The model under review builds one solid part; all positions refer to its coordinate system, in mm. Give positions to 0.01 mm unless a question says otherwise; leave off trailing zeros. Loops run counter-clockwise (first coordinate to the right, second up) from the corner with the lowest first, then second, coordinate; pieces in that order, holes last. Notation, with made-up numbers: M 65.5,37 L 122.5,37 A20 ccw 122.5,62 Z; hole C 81.5,52.5 d6. An arc over 180 degrees is marked long. One line per item, written item: value. Start each with the question number.
Q1. We need section B-B on z = -15377.5. Write out the cut boundary in (x, y).
Q2. To check wall thickness, follow line 1 along Z through (x, y) = (-9686, 2.5); line 2 along Z through (x, y) = (-9702, 3.1); line 3 along X through (y, z) = (2.9, -15375). State the ranges of each line that lie inside material, in increasing order. Write a range as from..to.
Q3. We need section A-A on y = 2.75. Write out the cut boundary in (x, z), plus the area to 3 significant figures.
Q4. We need section C-C on z = -15394. Write out the cut boundary in (x, y).
Q5. For pin 1 (1 mm diameter, centred on y = 2, z = -15392.5, fed in from +X); pin 2 (2 mm diameter, centred on x = -9630, y = 1.5, fed in from +Z), all flat-tipped, find the tip position at first contact; note any pin that passes through.
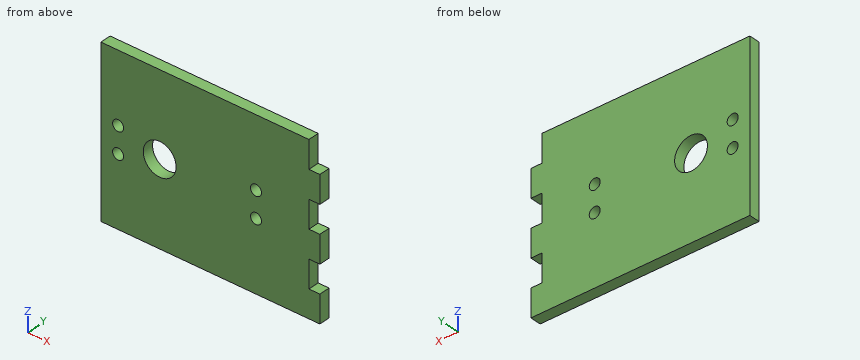
```python
from build123d import *

# Parameters (mm, degrees)
SKETCH1_R           = 6
SKETCH1_R_2         = 2
BOSS_EXTRUDE1_DEPTH = 4


with BuildPart() as part:
    # Sketch1 → Boss-Extrude1 (new body)
    with BuildSketch(Plane(origin=(0, 0, 0), x_dir=(1, 0, 0), z_dir=(0, 1, 0))):
        Polygon((-9707.918733038, 15348.509362373), (-9631.918733038, 15348.509362373), (-9631.918733038, 15358.505402083), (-9627.918733038, 15358.505402083), (-9627.918733038, 15368.509362373), (-9631.918733038, 15368.509362373), (-9631.918733038, 15378.509362373), (-9627.918733038, 15378.509362373), (-9627.918733038, 15388.509362373), (-9631.918733038, 15388.509362373), (-9631.918733038, 15398.509362373), (-9627.918733038, 15398.509362373), (-9627.918733038, 15408.509362373), (-9707.918733038, 15408.509362373), align=None)
        with Locations((-9686.434317231, 15378.509362373)):
            Circle(SKETCH1_R, mode=Mode.SUBTRACT)
        with Locations((-9651.234317231, 15383.259362373)):
            Circle(SKETCH1_R_2, mode=Mode.SUBTRACT)
        with Locations((-9651.234317231, 15373.759362373)):
            Circle(SKETCH1_R_2, mode=Mode.SUBTRACT)
        with Locations((-9701.634317231, 15373.759362373)):
            Circle(SKETCH1_R_2, mode=Mode.SUBTRACT)
        with Locations((-9701.634317231, 15383.259362373)):
            Circle(SKETCH1_R_2, mode=Mode.SUBTRACT)
    extrude(amount=BOSS_EXTRUDE1_DEPTH)


solid = part.part
```
Solved:
1. outline: M -9707.92,0 L -9692.35,0 L -9692.35,4 L -9707.92,4 Z; M -9680.52,0 L -9631.92,0 L -9631.92,4 L -9680.52,4 Z
2. line 1: -15408.51..-15384.49, -15372.53..-15348.51
2. line 2: -15408.51..-15385.23, -15381.29..-15375.73, -15371.79..-15348.51
2. line 3: -9707.92..-9703.2, -9700.07..-9691.3, -9681.57..-9652.8, -9649.67..-9631.92
3. outline: M -9707.92,-15408.51 L -9627.92,-15408.51 L -9627.92,-15398.51 L -9631.92,-15398.51 L -9631.92,-15388.51 L -9627.92,-15388.51 L -9627.92,-15378.51 L -9631.92,-15378.51 L -9631.92,-15368.51 L -9627.92,-15368.51 L -9627.92,-15358.51 L -9631.92,-15358.51 L -9631.92,-15348.51 L -9707.92,-15348.51 Z; hole C -9701.63,-15383.26 d4; hole C -9701.63,-15373.76 d4; hole C -9686.43,-15378.51 d12; hole C -9651.23,-15383.26 d4; hole C -9651.23,-15373.76 d4
3. area: 4,520 mm2
4. outline: M -9707.92,0 L -9631.92,0 L -9631.92,4 L -9707.92,4 Z
5. pin 1: x = -9631.92
5. pin 2: z = -15358.51
